Verification items for the finished model (mm, model axes). Round coordinates to 2 decimals unless told otherwise and drop trailing zeros. Write each loop counter-clockwise with the first axis right and the second up, starting at its lowest first coordinate (ties: lowest second). Pieces come first, ordered by that corner, then holes. Notation, with made-up numbers: (69, 85.5) - (127, 85.5) arc R9 ccw to (127, 93.5) - close; hole circle Ø11 at (-10, 81). An arc over 180 degrees is marked (long way). Write each question's results on one line, items separated by ' | '.
```python
from build123d import *

# Parameters (mm, degrees)
BOSS_EXTRUDE1_DEPTH = 50
FILLET1_R           = 2


with BuildPart() as part:
    # Sketch1 → Boss-Extrude1 (new body)
    with BuildSketch(Plane.XY):
        Polygon((0, 0), (-20, 0), (-30.606601718, -16.955824958), (-30.606601718, -46.955824958), (-20, -57.562426676), (0, -57.562426676), (10.606601718, -46.955824958), (10.606601718, -16.955824958), align=None)
    extrude(amount=BOSS_EXTRUDE1_DEPTH)

    # Fillet1
    fillet1_edges = [part.edges().sort_by_distance(p)[0] for p in [
        (-30.606601718, -31.955824958, 0),
        (-25.303300859, -8.477912479, 0),
        (-10, 0, 0),
        (5.303300859, -8.477912479, 0),
        (-25.303300859, -8.477912479, 50),
        (10.606601718, -16.955824958, 25),
        (10.606601718, -46.955824958, 25),
        (0, -57.562426676, 25),
        (-20, -57.562426676, 25),
        (-30.606601718, -46.955824958, 25),
        (-30.606601718, -16.955824958, 25),
        (-20, 0, 25),
        (0, 0, 25),
        (-30.606601718, -31.955824958, 50),
        (-25.303300859, -52.259125817, 50),
        (-10, -57.562426676, 50),
        (5.303300859, -52.259125817, 50),
        (10.606601718, -31.955824958, 50),
        (5.303300859, -8.477912479, 50),
        (10.606601718, -31.955824958, 0),
        (-10, 0, 50),
        (5.303300859, -52.259125817, 0),
        (-10, -57.562426676, 0),
        (-25.303300859, -52.259125817, 0),
    ]]
    fillet(fillet1_edges, radius=FILLET1_R)


solid = part.part
```
(1) Section check A-A (z = 6.5). Record the cut outline in (x, y), plus the area to 3 significant figures.
Answer:
outline: (-30.61, -46.13) arc R2 ccw to (-30.02, -47.54) - (-20.59, -56.98) arc R2 ccw to (-19.17, -57.56) - (-0.83, -57.56) arc R2 ccw to (0.59, -56.98) - (10.02, -47.54) arc R2 ccw to (10.61, -46.13) - (10.61, -17.53) arc R2 ccw to (10.3, -16.47) - (0.59, -0.94) arc R2 ccw to (-1.11, 0) - (-18.89, 0) arc R2 ccw to (-20.59, -0.94) - (-30.3, -16.47) arc R2 ccw to (-30.61, -17.53) - close | area: 2,080 mm2
(2) Thickness scan on L1, parallel to X at y = -15.5, z = 17.5; L2, parallel to Y at x = -28, z = 23.5; L3, parallel to Y at x = 5, z = 22. Record the ranges inside material, lowest first.
Answer:
L1: -29.7 to 9.7 | L2: -49.56 to -12.79 | L3: -52.56 to -7.99
(3) Go/stop test with flat-tipped pins: pin 1 Ø2 at (y, z) = (-15, 44) entering from +X; pin 2 Ø10 at (x, z) = (6.5, 22) entering from +Y; pin 3 Ø8 at (x, z) = (3.5, 13) entering from -Y. Record where each tip stops, or that it passes through.
Answer:
pin 1: x = 10.01 | pin 2: y = -2.4 | pin 3: y = -57.54
